For this review, use the dimensioned drawing (mm, ordinates from the lowest corner) and the shaded views. A direction names the side the tool comes from. Coordinates: 2 decimals unless noted, no trailing zeros. Loops run counter-clockwise (first coordinate to the right, second up) from the corner with the lowest first, then second, coordinate; pieces in that order, holes last. Notation, with made-up numbers: (73.25, 86) - (81.25, 86) arc R11 cw to (81.25, 107) - close; hole circle Ø7 at (27, -10). An arc over 180 degrees is marked (long way). Answer in a Markdown table with one row per item. Add a question column.
(1) For the marked faces 4, 5, 6, 7 and 8, list the 3-axis set-ups (+Z, -Z, +X, -X, +Y, -Y) from which the entire face can be reached by the end or side of a thin tool; tool diameter is ignored.
(2) To check wall thickness, follow L1, parallel to Z at x = 6, y = 165 (1 decimal); L2, parallel to Z at x = 44, y = 161 (1 decimal); L3, parallel to Z at x = 19, y = 67. State the ranges of each line that lie inside material, in increasing order. Write a range as [from, to].
(3) We need section D-D, the plane y = 16. Write out the cut boundary in (x, z).
(4) We need section A-A, the plane z = 51.5. Write out the cut boundary in (x, y) (1 decimal), plus the area to 3 significant figures.
(5) The part is to be moulded in two halves that separate along Z. For the marked faces 1, 2 and 3, say which applies: released by +Z, released by -Z, zero draft, split by the parting line, or undercut.
(6) Clearance check with flat-ended pins moving along their axes: pin 1 (1.5 mm diameter, centred on x = 22.5, y = 117, fed in from -Z); pin 2 (6 mm diameter, centred on x = 5.5, y = 33, fed in from +Z); pin 3 (2 mm diameter, centred on x = 18, y = 33, fed in from +Z) (1 decimal). State where each tip first meets the part, or that it passes through.
(7) We need section C-C, the plane y = 150. Write out the cut boundary in (x, z) (1 decimal), plus the area to 3 significant figures.
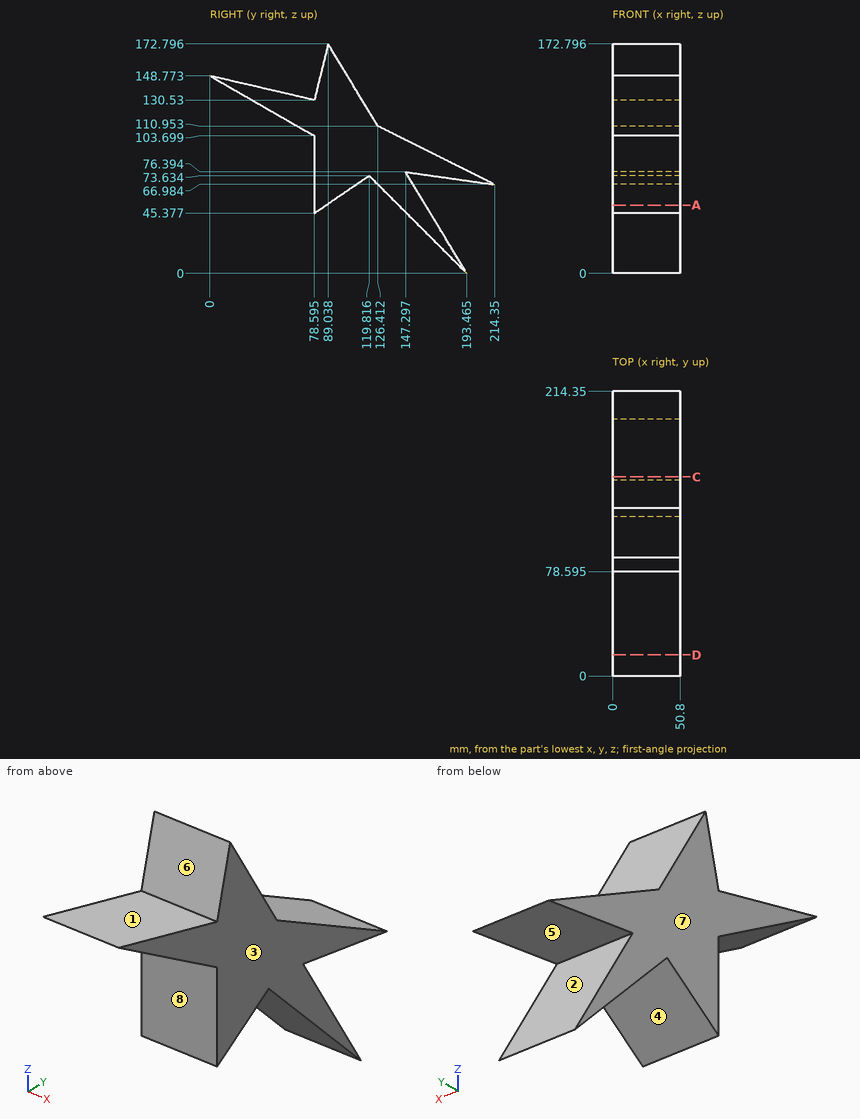
Responses:
| question | item | result |
|---|---|---|
| 1 | face 4 | -Z, +X, -X |
| 1 | face 5 | +X, -X |
| 1 | face 6 | +Z, +X, -X |
| 1 | face 7 | +Z, -Z, -X, +Y, -Y |
| 1 | face 8 | -Z, +X, -X, -Y |
| 2 | L1 | z = [28.5, 47.1], [73.9, 91.7] |
| 2 | L2 | z = [32.5, 53.7], [74.5, 93.7] |
| 2 | L3 | z = [110.35, 133.22] |
| 3 | outline | (0, 139.6) - (50.8, 139.6) - (50.8, 145.06) - (0, 145.06) - close |
| 4 | outline | (0, 78.6) - (50.8, 78.6) - (50.8, 87.5) - (0, 87.5) - close; (0, 142) - (50.8, 142) - (50.8, 162.3) - (0, 162.3) - close |
| 4 | area | 1,490 mm2 |
| 5 | face 1 | released by +Z |
| 5 | face 2 | undercut |
| 5 | face 3 | zero draft |
| 6 | pin 1 | stops at z = 71.19 |
| 6 | pin 2 | stops at z = 141.81 |
| 6 | pin 3 | stops at z = 141.3 |
| 7 | outline | (0, 43.5) - (50.8, 43.5) - (50.8, 71.9) - (0, 71.9) - close; (0, 76) - (50.8, 76) - (50.8, 99.2) - (0, 99.2) - close |
| 7 | area | 2,620 mm2 |
